```python
from build123d import *

# Parameters (mm, degrees)
F0_W     = 10
F0_H     = 6.09
F1_DEPTH = 10.9
F2_W     = 10.9
F2_H     = 2.09
F3_DEPTH = 25
F5_DEPTH = 12
F6_W     = 10
F6_H     = 2
F7_DEPTH = 25


with BuildPart() as f1:
    # F0 (on Right) → F1 (new body)
    with BuildSketch(Plane.YZ):
        with Locations((5, 3.045)):
            Rectangle(F0_W, F0_H)
    extrude(amount=F1_DEPTH)

    # F2 (on face) → F3 (cut)
    with BuildSketch(Plane.XZ):
        with Locations((5.45, 5.045)):
            Rectangle(F2_W, F2_H)
        Polygon((0, 0), (2.72, 0), (0, 2.48), align=None)
        Polygon((8.18, 0), (10.9, 0), (10.9, 2.48), align=None)
    extrude(amount=-F3_DEPTH, mode=Mode.SUBTRACT)

    # F4 (on face) → F5 (join)
    with BuildSketch(Plane.XY.offset(4)):
        Polygon((8.15, 10), (5.45, 10), (2.75, 10), (2.75, 0), (8.15, 0), align=None)
    extrude(amount=F5_DEPTH)

    # F6 (on face) → F7 (cut)
    with BuildSketch(Plane.YZ.offset(8.15)):
        with BuildLine():
            Line((3, 10), (7, 10))
            ThreePointArc((7, 10), (5, 12), (3, 10))
        make_face()
        with BuildLine():
            ThreePointArc((3, 10), (5, 8), (7, 10))
            Line((7, 10), (3, 10))
        make_face()
        with Locations((5, 15)):
            Rectangle(F6_W, F6_H)
    extrude(amount=-F7_DEPTH, mode=Mode.SUBTRACT)


solid = f1.part
```
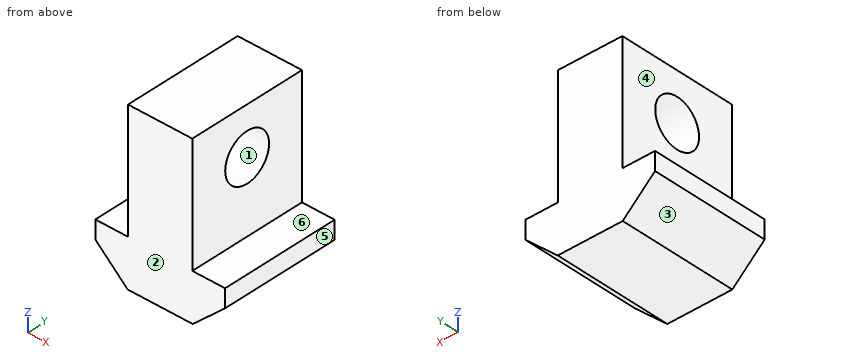
Geometry check sheet. Reference: the model listing, model coordinates, mm. Face numbers are marked on the shaded views. A direction names the side the tool comes from. Give positions to 0.01 mm unless a question says otherwise; leave off trailing zeros. Loops run counter-clockwise (first coordinate to the right, second up) from the corner with the lowest first, then second, coordinate; pieces in that order, holes last. Notation, with made-up numbers: M 58,82.25 L 101,82.25 A12 ccw 101,102.25 Z; hole C 79,72.5 d6. An arc over 180 degrees is marked long. Write item = value, one per line.
(1) Release check for a two-part mould opening along Y. For the marked faces 1, 2 and 3 record: released by +Y, released by -Y, zero draft, split by the parting line, or undercut.
Answer below:
face_1 = undercut
face_2 = released by -Y
face_3 = zero draft
(2) Sectioned sample at A-A, the plane y = 5. Record the cut outline in (x, z).
Answer below:
outline = M 0,2.48 L 2.72,0 L 8.18,0 L 10.9,2.48 L 10.9,4 L 8.15,4 L 8.15,8 L 2.75,8 L 2.75,4 L 0,4 Z; M 2.75,12 L 8.15,12 L 8.15,14 L 2.75,14 Z
(3) Sectioned sample at D-D, the plane y = 2. Record the cut outline in (x, z), plus the area to 3 significant figures.
Answer below:
outline = M 0,2.48 L 2.72,0 L 8.18,0 L 10.9,2.48 L 10.9,4 L 8.15,4 L 8.15,14 L 2.75,14 L 2.75,4 L 0,4 Z
area = 90.9 mm2
(4) Gauge pin test, flat ends, axial feed: pin 1 Ø0.8 at (x, y) = (9, 6.5) entering from +Z; pin 2 Ø3 at (y, z) = (6.5, 10.5) entering from -X; pin 3 Ø1.5 at (y, z) = (3, 9.5) entering from +X. Record the tip position at first contact, or that the pin passes through.
Answer below:
pin_1 = 4
pin_2 = 2.75
pin_3 = 8.15
(5) Material ranges on line 1 (Y direction, x = 6.25, z = 10); line 2 (Z direction, x = 4.6, y = 5); line 3 (X direction, y = 7, z = 12.25), recorded low to high. Write a range as [from, to].
Answer below:
line_1 = [0, 3], [7, 10]
line_2 = [0, 8], [12, 14]
line_3 = [2.75, 8.15]
(6) Sectioned sample at B-B, the plane z = 10. Record the cut outline in (x, y).
Answer below:
outline = M 2.75,0 L 8.15,0 L 8.15,3 L 2.75,3 Z; M 2.75,7 L 8.15,7 L 8.15,10 L 2.75,10 Z
(7) Sectioned sample at C-C, the plane x = 7. Record the cut outline in (y, z), plus the area to 3 significant figures.
Answer below:
outline = M 0,0 L 10,0 L 10,14 L 0,14 Z; hole C 5,10 d4
area = 127 mm2
(8) Tool access check on the marked faces 4, 5 and 6. Record the directions out of +Z, -Z, +X, -X, +Y, -Y that give a thin tool (end or side, any length) a straight path to the whole face; none if there is none.
Answer below:
face_4 = +Z, -X, +Y, -Y
face_5 = +Z, -Z, +X, +Y, -Y
face_6 = +Z, +X, +Y, -Y
